Can you work these out from the model? Positions are in its coordinate system, mm. A direction names the side the tool comes from. Coordinates: 2 decimals unless noted, no trailing zeros. Write each loop counter-clockwise with the first axis right and the second up, starting at its lowest first coordinate (ties: lowest second). Pieces come first, ordered by that corner, then holes. Notation, with made-up numbers: (48.5, -40) -> (96.5, -40) arc R19 ccw to (96.5, -5) -> close; hole circle Ø3 at (-18, 31). An arc over 180 degrees is marked (long way). Use one line per item in the form item = value.
```python
from build123d import *

# Parameters (mm, degrees)
SKETCH_1_W      = 92
SKETCH_1_H      = 56
SKETCH_1_W_2    = 4
SKETCH_1_H_2    = 18
SKETCH_1_W_3    = 20
SKETCH_1_H_3    = 4
EXTRUDE_1_DEPTH = 4


with BuildPart() as part:
    # 草图1 → 凸台-拉伸1 (new body)
    with BuildSketch(Plane(origin=(0, 0, 0), x_dir=(1, 0, 0), z_dir=(0, 1, 0))):
        with Locations((46, 28)):
            Rectangle(SKETCH_1_W, SKETCH_1_H)
        with Locations((-2, 9)):
            Rectangle(SKETCH_1_W_2, SKETCH_1_H_2)
        with Locations((-2, 47)):
            Rectangle(SKETCH_1_W_2, SKETCH_1_H_2)
        with Locations((46, -2)):
            Rectangle(SKETCH_1_W_3, SKETCH_1_H_3)
        with Locations((94, 9)):
            Rectangle(SKETCH_1_W_2, SKETCH_1_H_2)
        with Locations((94, 47)):
            Rectangle(SKETCH_1_W_2, SKETCH_1_H_2)
    extrude(amount=EXTRUDE_1_DEPTH)


solid = part.part
```
Q1. Suppose I cut it at C-C (x = 68). Write out the boundary of the cut face in (y, z).
Return value:
outline = (0, -56) -> (4, -56) -> (4, 0) -> (0, 0) -> close
Q2. Suppose I cut it at A-A (y = 2.35). Write out the boundary of the cut face in (x, z).
Return value:
outline = (-4, -56) -> (96, -56) -> (96, -38) -> (92, -38) -> (92, -18) -> (96, -18) -> (96, 0) -> (56, 0) -> (56, 4) -> (36, 4) -> (36, 0) -> (-4, 0) -> (-4, -18) -> (0, -18) -> (0, -38) -> (-4, -38) -> close
Q3. Suppose I cut it at B-B (z = -31). Write out the boundary of the cut face in (x, y).
Return value:
outline = (0, 0) -> (92, 0) -> (92, 4) -> (0, 4) -> close
Q4. For faces 4 (the flat face through (56, 2, 2)), 5 (the flat face through (-2, 2, -18)), 6 (the flat face through (92, 2, -28)), 7 (the flat face through (16, 2, 0)), which set-ups out of +Z, -Z, +X, -X, +Y, -Y let a thin tool reach every point of the face, with its end or its side?
Return value:
face_4 = +Z, +X, +Y, -Y
face_5 = -X, +Y, -Y
face_6 = +X, +Y, -Y
face_7 = +Z, -X, +Y, -Y
Q5. Will these pins go through, and if not, where does the flat tip stop? pin 1 (2 mm diameter, centred on x = 85.5, y = 1.5, fed in from +Z); pin 2 (1.2 mm diameter, centred on y = 3, z = 3, fed in from +X); pin 3 (2 mm diameter, centred on y = 2, z = -31.5, fed in from -X); pin 4 (10 mm diameter, centred on x = 18, z = -49, fed in from -Y).
Return value:
pin_1 = 0
pin_2 = 56
pin_3 = 0
pin_4 = 0
Q6. Thinking about a two-plate mould opening in Z: for faces 1 (the flat face through (76, 2, 0)), 2 (the flat face through (94, 2, -18)), 3 (the flat face through (47, 2, -56)), which applies, released by +Z, released by -Z, zero draft, split by the parting line, or undercut?
Return value:
face_1 = released by +Z
face_2 = undercut
face_3 = released by -Z
Q7. If I drill on line 1 (Z direction, x = 84, y = 3.55); line 2 (X direction, y = 1.35, z = 1.5); line 3 (X direction, y = 3, z = -31), over which ranges is the centre line in solid material (lowest first)? Write a range as from..to.
Return value:
line_1 = -56..0
line_2 = 36..56
line_3 = 0..92
